Answer from the drawing. Dimensions are ordinates in mm from the lowest x, y and z of the part. A direction names the side the tool comes from. Give positions to 0.01 mm unless a question says otherwise; leave off trailing zeros. Loops run counter-clockwise (first coordinate to the right, second up) from the corner with the lowest first, then second, coordinate; pieces in that order, holes last. Notation, with made-up numbers: (65, 10) - (82, 10) arc R15 cw to (82, 21) - close; hole circle Ø11 at (13.25, 16). An arc over 180 degrees is marked (long way). Answer as CSV lines item,"result". Start each with the question number.
1) A cutting plane is placed at A-A (z = 524). Determine the outline of the cut face in (x, y).
2) A cutting plane is placed at C-C (y = 1068). Determine the outline of the cut face in (x, z), and give its area (3 significant figures).
3) Find the intervals of material crossed by line 1 along Y through (x, z) = (729.5, 943.5); line 2 along Y through (x, z) = (1317, 676); line 3 along Z through (x, y) = (1083, 934.5), in increasing order.
4) For the marked faces 1 and 2, determine the directions among +Z, -Z, +X, -X, +Y, -Y from which every point of the face is accessible in a straight line to the end or side of a thin tool.
5) Flat-ended cylindrical pins translate along their axes: pin 1 (6 mm diameter, centred on x = 1116, z = 693.5, fed in from +Y); pin 2 (4 mm diameter, centred on x = 1192, z = 370, fed in from +Y). Find the tip coordinate at first contact, or state that the pin passes through.
6) A cutting plane is placed at D-D (z = 750). Determine the outline of the cut face in (x, y), and give its area (3 significant figures).
7) A cutting plane is placed at B-B (x = 800). Determine the outline of the cut face in (y, z), and give its area (3 significant figures).
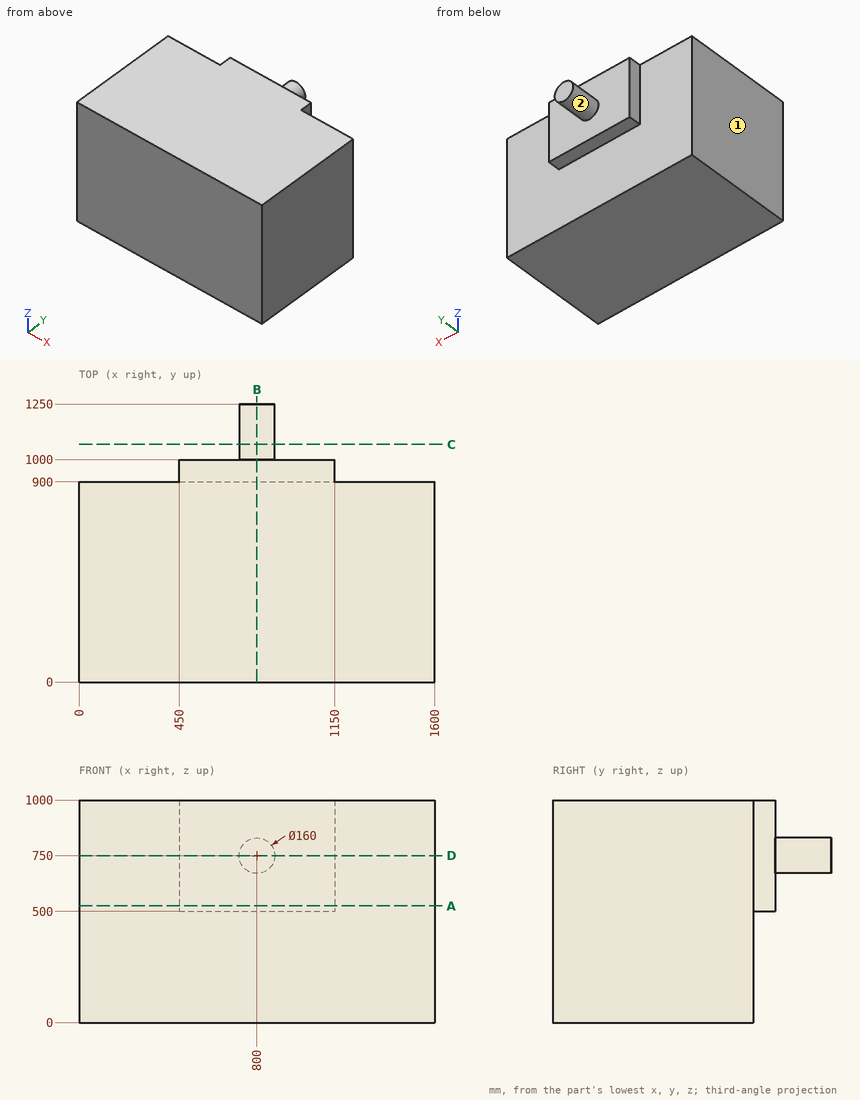
Ans:
1,outline,"(0, 0) - (1600, 0) - (1600, 900) - (1150, 900) - (1150, 1000) - (450, 1000) - (450, 900) - (0, 900) - close"
2,outline,"circle Ø160 at (800, 750)"
2,area,"20,100 mm2"
3,line 1,"0 to 1000"
3,line 2,"0 to 900"
3,line 3,"500 to 1000"
4,face 1,"+Z, -Z, -X, +Y, -Y"
4,face 2,"+Y"
5,pin 1,"y = 1000"
5,pin 2,"y = 900"
6,outline,"(0, 0) - (1600, 0) - (1600, 900) - (1150, 900) - (1150, 1000) - (880, 1000) - (880, 1250) - (720, 1250) - (720, 1000) - (450, 1000) - (450, 900) - (0, 900) - close"
6,area,"1,550,000 mm2"
7,outline,"(0, 0) - (900, 0) - (900, 500) - (1000, 500) - (1000, 670) - (1250, 670) - (1250, 830) - (1000, 830) - (1000, 1000) - (0, 1000) - close"
7,area,"990,000 mm2"
